The drawing under review shows one solid part. Ordinate dimensions are in mm from its lowest x, y, z. A direction names the side the tool comes from. Round coordinates to 2 decimals unless told otherwise and drop trailing zeros. Loops run counter-clockwise (first coordinate to the right, second up) from the corner with the lowest first, then second, coordinate; pieces in that order, holes last. Notation, with made-up numbers: (-36, 35) -> (-28, 35) arc R30 cw to (-28, 60) -> close; hole circle Ø8 at (58, 37.5). An arc over 180 degrees is marked (long way). Use a Markdown table: item, result. Add a question column.
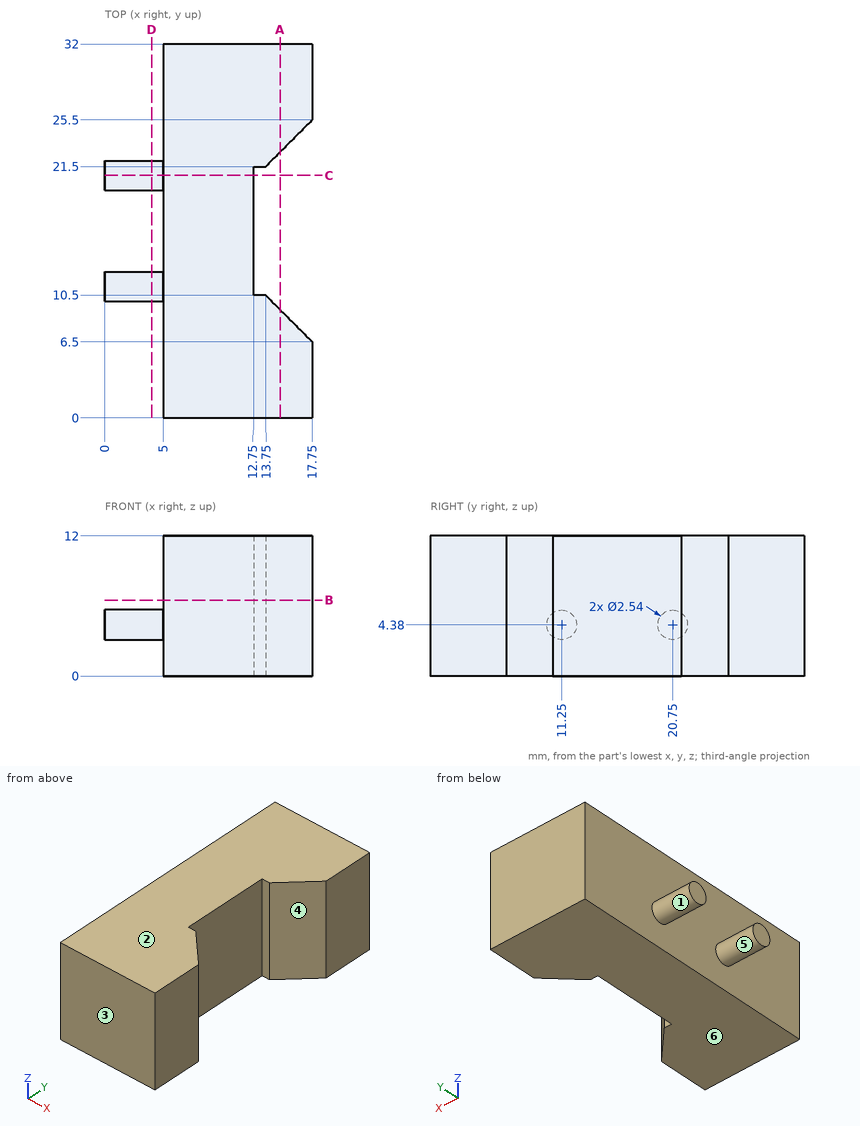
1. Consider section A-A on x = 15. State the section outline as (y, z) points.
2. Consider section B-B on z = 6.5. State the section outline as (x, y) points.
3. Consider section D-D on x = 4. State the section outline as (y, z) points.
4. Consider section C-C on y = 20.75. State the section outline as (x, z) points.
5. Mouldability with a two-part tool opening along Y and no side actions: class the marked faces 1, 2 and 3 as +Y half, -Y half, draft (parallel to the pull), parting line (faces both ways), or undercut.
6. To check wall thickness, follow probe 1 along X at (y, z) = (3.5, 8.25); probe 2 along Y at (x, z) = (13.5, 8.5); probe 3 along X at (y, z) = (13.5, 10). State the ranges of each line that lie inside material, in increasing order. Write a range as from..to.
7. For the marked faces 4, 5 and 6, list the 3-axis set-ups (+Z, -Z, +X, -X, +Y, -Y) from which the entire face can be reached by the end or side of a thin tool; tool diameter is ignored.
Verdict:
| question | item | result |
|---|---|---|
| 1 | outline | (0, 0) -> (9.25, 0) -> (9.25, 12) -> (0, 12) -> close; (22.75, 0) -> (32, 0) -> (32, 12) -> (22.75, 12) -> close |
| 2 | outline | (5, 0) -> (17.75, 0) -> (17.75, 6.5) -> (13.75, 10.5) -> (12.75, 10.5) -> (12.75, 21.5) -> (13.75, 21.5) -> (17.75, 25.5) -> (17.75, 32) -> (5, 32) -> close |
| 3 | outline | circle Ø2.54 at (11.25, 4.38); circle Ø2.54 at (20.75, 4.38) |
| 4 | outline | (0, 3.11) -> (5, 3.11) -> (5, 0) -> (12.75, 0) -> (12.75, 12) -> (5, 12) -> (5, 5.65) -> (0, 5.65) -> close |
| 5 | face 1 | undercut |
| 5 | face 2 | draft |
| 5 | face 3 | -Y half |
| 6 | probe 1 | x = 5..17.75 |
| 6 | probe 2 | y = 0..10.5, 21.5..32 |
| 6 | probe 3 | x = 5..12.75 |
| 7 | face 4 | +Z, -Z, +X |
| 7 | face 5 | -X |
| 7 | face 6 | -Z, +X, -X, +Y, -Y |
